Check sheet for the modelled part. Datum: model origin and axes. Units: mm. Coordinates: 2 decimals unless noted, no trailing zeros. Loops run counter-clockwise (first coordinate to the right, second up) from the corner with the lowest first, then second, coordinate; pieces in that order, holes last. Notation, with made-up numbers: (-24, 51.5) - (34, 51.5) arc R29 ccw to (34, 77.5) - close; hole circle Ø9 at (-23.75, 10.5). An arc over 180 degrees is marked (long way). Write each question's results on one line, items separated by ' | '. Start each with the question number.
1. Gauge pin test, flat ends, axial feed: P1, Ø2, axis at x = 6, y = -31.8, coming from the -Z side; P2, Ø0.5, axis at x = 1.5, z = 0, coming from the +Y side; P3, Ø1.4, axis at x = 6, y = 31.8, coming from the -Z side; P4, Ø8, axis at x = 9.5, y = -11.5, coming from the +Z side. Record the tip position at first contact, or that the pin passes through.
2. Cross-section at C-C (y = -13.5). Record the cut outline in (x, z), and give its area (3 significant figures).
3. Thickness scan on line 1 (Y direction, x = 6, z = 0.2); line 2 (Z direction, x = 75.5, y = 20); line 3 (X direction, y = -44, z = 0.35). Record the ranges inside material, lowest first. Write a range as [from, to].
4. Cross-section at A-A (z = 0). Record the cut outline in (x, y), and give its area (3 significant figures).
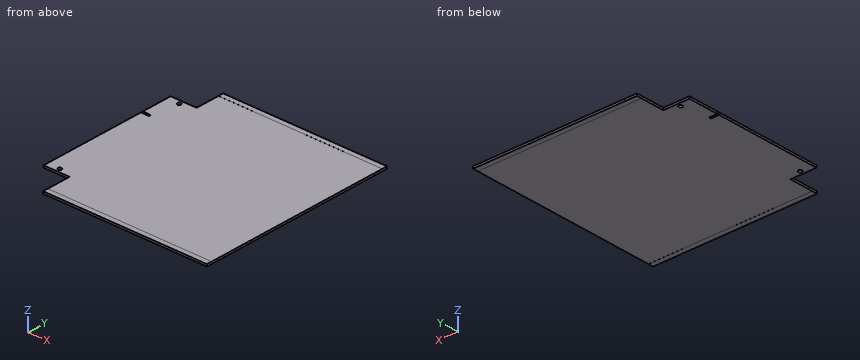
Autodesk Inventor part; units mm, degrees
ref_plane "YZ Plane" through (0, 0, 0) normal (1, 0, 0) x (0, 1, 0)
ref_plane "XZ Plane" through (0, 0, 0) normal (0, 1, 0) x (-1, 0, 0)
ref_plane "XY Plane" through (0, 0, 0) normal (0, 0, 1) x (1, 0, 0)
sketch "Sketch1" plane through (0, 0, 0) normal (0, 0, 1) x (1, 0, 0)
  line L0 (0, 33.8) -> (12.5, 33.8)
  line L1 (12.5, 33.8) -> (12.5, 47.9)
  line L2 (12.5, 47.9) -> (91.4, 47.9)
  line L3 (91.4, 47.9) -> (91.4, -47.9)
  line L4 (91.4, -47.9) -> (12.5, -47.9)
  line L5 (12.5, -47.9) -> (12.5, -33.8)
  line L6 (12.5, -33.8) -> (0, -33.8)
  line L7 (0, -33.8) -> (0, 33.8)
  line L8 (-4.5, 48) -> (91.5, 48) construction
  line L9 (91.5, 48) -> (91.5, -48) construction
  line L10 (91.5, -48) -> (-4.5, -48) construction
  line L11 (-4.5, -48) -> (-4.5, 48) construction
  line L12 (-4.4, 47.9) -> (-3.4, 47.9) construction
  line L13 (-3.4, 47.9) -> (-3.4, -47.9) construction
  line L14 (-3.4, -47.9) -> (-4.4, -47.9) construction
  line L15 (-4.4, -47.9) -> (-4.4, 47.9) construction
  point P0 (0, 0)
  point P1 (0, 0)
  point P2 (-4.5, 0)
  dimension "d0" = 67.6
  dimension "d1" = 95.8
  dimension "d2" = 91.4
  dimension "d3" = 12.5
  dimension "d20" = 96
  dimension "d21" = 96
  dimension "d22" = 0.1
  dimension "d23" = 0.1
  dimension "d24" = 1
  dimension "d25" = 0.1
  dimension "d26" = 3.4
extrude "Extrusion1" add sketch "Sketch1" along normal mid plane 1
sketch "Sketch2" plane through (0, 0, 0.5) normal (0, 0, 1) x (1, 0, 0)
  line L0 (12.5, 33.8) -> (0, 33.8)
  line L1 (0, 33.8) -> (0, -33.8)
  line L2 (0, -33.8) -> (12.5, -33.8)
  line L3 (12.5, -33.8) -> (12.5, -47.9)
  line L4 (12.5, -47.9) -> (91.4, -47.9)
  line L5 (91.4, -47.9) -> (91.4, 47.9)
  line L6 (91.4, 47.9) -> (12.5, 47.9)
  line L7 (12.5, 47.9) -> (12.5, 33.8)
  line L8 (91.4, -47.9) -> (91.4, 47.9)
  line L9 (12.5, 47.9) -> (91.4, 47.9)
  line L10 (91.4, 47.9) -> (91.4, 45.4)
  line L11 (91.4, 45.4) -> (12.5, 45.4)
  line L12 (12.5, 45.4) -> (12.5, 47.9)
  line L13 (91.4, -47.9) -> (12.5, -47.9)
  line L14 (12.5, -47.9) -> (12.5, -45.4)
  line L15 (12.5, -45.4) -> (91.4, -45.4)
  line L16 (91.4, -45.4) -> (91.4, -47.9)
  point P0 (0, 0)
  dimension "d6" = 2.5
  dimension "d27" = 90.8
extrude "Extrusion2" add sketch "Sketch2" along normal blind 0.01 contours L7 L6 L5 L11 | L5 L4 L3 L15
mirror "Mirror1" about plane through (0, 0, 0) normal (0, 0, 1) of "Extrusion2"
sketch "Sketch3" plane through (0, 0, 0.5) normal (0, 0, 1) x (1, 0, 0)
  circle A0 centre (6, 31.8) radius 0.9
  circle A1 centre (6, -31.8) radius 0.9
  point P0 (0, 0)
  dimension "d9" = 1.8
  dimension "d10" = 6
  dimension "d11" = 31.8
  dimension "d12" = 31.8
extrude "Extrusion3" cut sketch "Sketch3" against normal through all
sketch "Sketch4" plane through (0, 0, 0.5) normal (0, 0, 1) x (1, 0, 0)
  circle A0 centre (6, 31.8) radius 0.9
  circle A1 centre (6, -31.8) radius 0.9
  line L0 (12.5, -45.4) -> (91.4, -45.4)
  line L1 (91.4, -45.4) -> (91.4, 45.4)
  line L2 (91.4, 45.4) -> (12.5, 45.4)
  line L3 (12.5, 45.4) -> (12.5, 33.8)
  line L4 (12.5, 33.8) -> (0, 33.8)
  line L5 (0, 33.8) -> (0, -33.8)
  line L6 (0, -33.8) -> (12.5, -33.8)
  line L7 (12.5, -33.8) -> (12.5, -45.4)
  line L8 (0, 18.95) -> (3.5, 18.95)
  arc A2 (3.5, 17.95) -> (3.5, 18.95) centre (3.5, 18.45) ccw
  line L9 (3.5, 17.95) -> (0, 17.95)
  point P0 (0, 0)
  dimension "d15" = 17.95
  dimension "d16" = 3.5
  dimension "d17" = 1
extrude "Extrusion4" cut sketch "Sketch4" against normal through all contours L5 L8 A2 L9
equation "\"d23\" = d22"
equation "\"d25\" = d22"
properties part number "RCS_PCB" material "Epoxy Resin"
Established:
1) P1: z = -0.5 | P2: y = 33.8 | P3: through | P4: z = 0.5
2) outline: (0, -0.5) - (91.4, -0.5) - (91.4, 0.5) - (0, 0.5) - close | area: 91.4 mm^2
3) line 1: [-33.8, -32.7], [-30.9, 30.9], [32.7, 33.8] | line 2: [-0.5, 0.5] | line 3: [12.5, 91.4]
4) outline: (0, -33.8) - (12.5, -33.8) - (12.5, -47.9) - (91.4, -47.9) - (91.4, 47.9) - (12.5, 47.9) - (12.5, 33.8) - (0, 33.8) - (0, 18.95) - (3.5, 18.95) arc R0.5 cw to (3.5, 17.95) - (0, 17.95) - close; hole circle Ø1.8 at (6, -31.8); hole circle Ø1.8 at (6, 31.8) | area: 8,390 mm^2
